from build123d import *

# Parameters (mm, degrees)
SKETCH1_R   = 15.175
SKETCH1_R_2 = 12
SKETCH6_W   = 2.65
SKETCH6_H   = 15.175


with BuildPart() as part:
    # Sweep1: sweep along a path in Sketch3
    with BuildLine(Plane(origin=(0, 0, 0), x_dir=(0, 0, -1), z_dir=(1, 0, 0))) as sweep1_path:
        Line((0, 0), (40, 0))
        ThreePointArc((40, 0), (54.142135624, -5.857864376), (60, -20))
        Line((60, -20), (60, -60))
    # Sketch1 → Sweep1 (sweep)
    with BuildSketch(Plane.XY):
        Circle(SKETCH1_R)
        Circle(SKETCH1_R_2, mode=Mode.SUBTRACT)
    sweep(path=sweep1_path.line)

    # Sketch6 → M5 Clearance Hole1 (revolve, cut)
    with BuildSketch(Plane(origin=(0, 0, -15), x_dir=(0, 0, 1), z_dir=(0, 1, 0))):
        with Locations((1.325, 7.5875)):
            Rectangle(SKETCH6_W, SKETCH6_H)
    m5_clearance_hole1 = revolve(axis=Axis((-6.35, 0, -15), (1, 0, 0)), mode=Mode.SUBTRACT)

    # Mirror1: M5 Clearance Hole1 across plane
    add(m5_clearance_hole1.mirror(Plane(origin=(0, 0, 0), x_dir=(0, 0, 1), z_dir=(1, 0, 0))), mode=Mode.SUBTRACT)


solid = part.part
The listing builds one solid part. Answer for the finished solid, in the listing's coordinates (mm). A direction names the side the tool comes from. Coordinates: 2 decimals unless noted, no trailing zeros. Loops run counter-clockwise (first coordinate to the right, second up) from the corner with the lowest first, then second, coordinate; pieces in that order, holes last.
1) A tool of negligible diameter and unlimited length cuts with its end or side. For faces 1 (the face through (14.474, -4.558, -20.28)), 2 (the face through (-7, -60, -50)), from which of +Z, -Z, +X, -X, +Y, -Y can it reach the whole face along a straight path? Write none if from no direction.
2) Determine the mould class of faces 3 (the face through (10, -7, 0)), 4 (the face through (-2.601, -40.28, -71.715)), 5 (the face through (-3.29, -40.28, -74.814)) for opening direction Z: pulls with the +Z half, pulls with the -Z half, needs draft (parallel to the pull), parting line crosses it, or undercut.
3) Find section C-C on y = 0. Give the number of separate pieces and of enclosed holes in the cut face, then the cut area to 3 significant figures.
4) Flat-ended cylindrical pins translate along their axes: pin 1 Ø2 at (y, z) = (6, -25) entering from +X; pin 2 Ø14.5 at (x, z) = (0, -60) entering from +Y; pin 3 Ø1 at (x, z) = (2, -12) entering from -Y. Find the tip coordinate at first contact, or state that the pin passes through.
5) Find section B-B on z = -15. Write down the section's boundary in (x, y) (3 decimals).
6) Find section D-D on z = -27.5. Write down the section's boundary in (x, y) (3 decimals), then the cut area to 3 significant figures.
7) Find section A-A on x = 0. Write down the section's boundary in (y, z) (3 decimals).
8) Find the intervals of material crossed by L1, parallel to Y at x = 0, z = -17 (3 decimals); L2, parallel to Y at x = 8, z = -25; L3, parallel to Z at x = -6, y = -34.5, in increasing order.
Values:
1. face 1: +Z
1. face 2: +Z, -Z, +X, -X, -Y
2. face 3: pulls with the +Z half
2. face 4: undercut
2. face 5: parting line crosses it
3. separate pieces: 3
3. enclosed holes: 0
3. area: 456 mm2
4. pin 1: stops at x = 14.33
4. pin 2: stops at y = 12.78
4. pin 3: stops at y = -15.1
5. outline: (-14.942, -2.65) arc R15.175 ccw to (14.942, -2.65) - (11.704, -2.65) arc R12 cw to (-11.704, -2.65) - close; (-14.942, 2.65) - (-11.704, 2.65) arc R12 cw to (11.704, 2.65) - (14.942, 2.65) arc R15.175 ccw to start
6. outline: circle Ø30.35 at (0, 0); hole circle Ø24 at (0, 0)
6. area: 271 mm2
7. outline: (-60, -75.175) - (-20, -75.175) arc R35.175 ccw to (15.175, -40) - (15.175, 0) - (12, 0) - (12, -40) arc R32 cw to (-20, -72) - (-60, -72) - close; (-60, -48) - (-20, -48) arc R8 ccw to (-12, -40) - (-12, 0) - (-15.175, 0) - (-15.175, -40) arc R4.825 cw to (-20, -44.825) - (-60, -44.825) - close
8. L1: y = -15.175 to -12, 12 to 15.175
8. L2: y = -12.89 to -8.94, 8.94 to 12.89
8. L3: z = -73.94 to -70.39, -49.61 to -46.06
